from build123d import *

# Parameters (mm, degrees)
SKETCH1_W               = 88.9
SKETCH1_H               = 25.4
BOSS_EXTRUDE1_DEPTH     = 38.1
CUT_EXTRUDE1_REACH      = 40.1
F_3_8_CLEARANCE_HOLE1_D = 9.8044


with BuildPart() as part:
    # Sketch1 → Boss-Extrude1 (new body)
    with BuildSketch(Plane.XY):
        with Locations((0, 12.7)):
            Rectangle(SKETCH1_W, SKETCH1_H)
    extrude(amount=-BOSS_EXTRUDE1_DEPTH)

    # Sketch2 → Cut-Extrude1 (cut, up to next)
    with BuildSketch(Plane.XY, mode=Mode.PRIVATE) as cut_extrude1_sk1:
        with BuildLine():
            Line((-15.875, 25.4), (0, 25.4))
            Line((0, 25.4), (15.875, 25.4))
            Line((15.875, 25.4), (15.875, 24.13))
            Line((15.875, 24.13), (14.410694861, 24.13))
            Line((14.410694861, 24.13), (14.410694861, 22.86))
            Line((14.410694861, 22.86), (12.946389723, 22.86))
            Line((12.946389723, 22.86), (12.946389723, 21.59))
            Line((12.946389723, 21.59), (11.482084584, 21.59))
            Line((11.482084584, 21.59), (11.482084584, 20.32))
            Line((11.482084584, 20.32), (10.017779445, 20.32))
            Line((10.017779445, 20.32), (10.017779445, 19.05))
            Line((10.017779445, 19.05), (8.553474306, 19.05))
            Line((8.553474306, 19.05), (8.553474306, 17.78))
            Line((8.553474306, 17.78), (7.089169168, 17.78))
            Line((7.089169168, 17.78), (7.089169168, 16.51))
            Line((7.089169168, 16.51), (5.624864029, 16.51))
            Line((5.624864029, 16.51), (5.624864029, 15.24))
            Line((5.624864029, 15.24), (4.16055889, 15.24))
            ThreePointArc((4.16055889, 15.24), (0, 13.687108475), (-4.16055889, 15.24))
            Line((-4.16055889, 15.24), (-5.624864029, 15.24))
            Line((-5.624864029, 15.24), (-5.624864029, 16.51))
            Line((-5.624864029, 16.51), (-7.089169168, 16.51))
            Line((-7.089169168, 16.51), (-7.089169168, 17.78))
            Line((-7.089169168, 17.78), (-8.553474306, 17.78))
            Line((-8.553474306, 17.78), (-8.553474306, 19.05))
            Line((-8.553474306, 19.05), (-10.017779445, 19.05))
            Line((-10.017779445, 19.05), (-10.017779445, 20.32))
            Line((-10.017779445, 20.32), (-11.482084584, 20.32))
            Line((-11.482084584, 20.32), (-11.482084584, 21.59))
            Line((-11.482084584, 21.59), (-12.946389723, 21.59))
            Line((-12.946389723, 21.59), (-12.946389723, 22.86))
            Line((-12.946389723, 22.86), (-14.410694861, 22.86))
            Line((-14.410694861, 22.86), (-14.410694861, 24.13))
            Line((-14.410694861, 24.13), (-15.875, 24.13))
            Line((-15.875, 24.13), (-15.875, 25.4))
        make_face()
    cut_extrude1_tool1 = extrude(cut_extrude1_sk1.sketch, amount=-CUT_EXTRUDE1_REACH, mode=Mode.PRIVATE) & part.part
    add(cut_extrude1_tool1.solids().sort_by_distance((0, 20.970592, 0))[0], mode=Mode.SUBTRACT)

    # 3/8 Clearance Hole1 (through all)
    with Locations(Plane(origin=(0, 25.4, 0), x_dir=(1, 0, 0), z_dir=(0, 1, 0))):
        with Locations((-31.75, 19.05), (31.75, 19.05)):
            Hole(F_3_8_CLEARANCE_HOLE1_D / 2)


solid = part.part
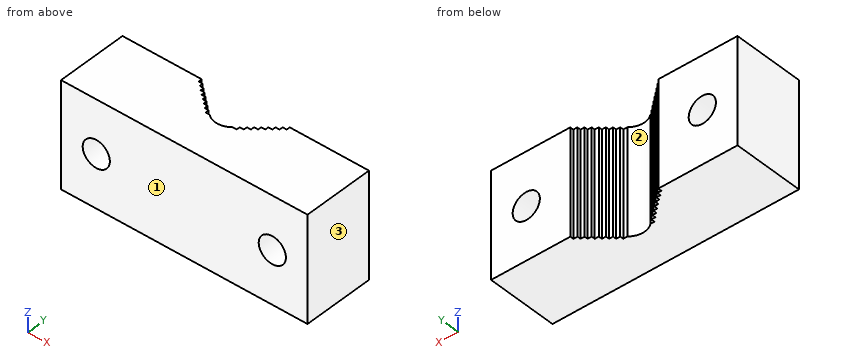
The model under review builds one solid part; all positions refer to its coordinate system, in mm. Face numbers are marked on the shaded views. Coordinates: 2 decimals unless noted, no trailing zeros. Loops run counter-clockwise (first coordinate to the right, second up) from the corner with the lowest first, then second, coordinate; pieces in that order, holes last. Notation, with made-up numbers: (45, 49) -> (49, 49) arc R29 ccw to (49, 85) -> close; hole circle Ø2 at (-3, -9.5). An arc over 180 degrees is marked (long way). Use a Markdown table: item, result. Add a question column.
1. Draft analysis for pull direction X (two halves, no side actions). For the marked faces 1, 2 and 3, state which applies: pulls with the +X half, pulls with the -X half, needs draft (parallel to the pull), parting line crosses it, or undercut.
2. Add section A-A on x = -31.75. Write out the cut boundary in (y, z).
3. Clearance check with flat-ended pins moving along their axes: pin 1 Ø0.7 at (x, z) = (-8, -10) entering from +Y; pin 2 Ø1.6 at (x, z) = (10.5, -17) entering from +Y. State where each tip first meets the part, or that it passes through.
4. To check wall thickness, follow line 1 (X direction, y = 11.5, z = -19.05); line 2 (X direction, y = 19.25, z = -19.05); line 3 (X direction, y = 17.25, z = -9.5). State the ranges of each line that lie inside material, in increasing order.
5. Add section C-C on z = -19.05. Give the number of separate pieces and of enclosed holes in the cut face, plus the area to 3 significant figures.
6. Add section D-D on x = 1.5. Write out the cut boundary in (y, z), plus the area to 3 significant figures.
7. Add section B-B on y = 12.5. Write out the cut boundary in (x, z).
Returned:
| question | item | result |
|---|---|---|
| 1 | face 1 | needs draft |
| 1 | face 2 | undercut |
| 1 | face 3 | pulls with the +X half |
| 2 | outline | (0, -38.1) -> (25.4, -38.1) -> (25.4, -23.95) -> (0, -23.95) -> close; (0, -14.15) -> (25.4, -14.15) -> (25.4, 0) -> (0, 0) -> close |
| 3 | pin 1 | stops at y = 17.78 |
| 3 | pin 2 | stops at y = 20.32 |
| 4 | line 1 | x = -44.45 to -36.65, -26.85 to 26.85, 36.65 to 44.45 |
| 4 | line 2 | x = -44.45 to -36.65, -26.85 to -10.02, 10.02 to 26.85, 36.65 to 44.45 |
| 4 | line 3 | x = -44.45 to -7.09, 7.09 to 44.45 |
| 5 | separate pieces | 3 |
| 5 | enclosed holes | 0 |
| 5 | area | 1,530 mm² |
| 6 | outline | (0, -38.1) -> (13.87, -38.1) -> (13.87, 0) -> (0, 0) -> close |
| 6 | area | 528 mm² |
| 7 | outline | (-44.45, -38.1) -> (44.45, -38.1) -> (44.45, 0) -> (-44.45, 0) -> close; hole circle Ø9.8 at (-31.75, -19.05); hole circle Ø9.8 at (31.75, -19.05) |
